Geometry: final body of the model. Coordinates: model frame, mm. Give positions to 0.01 mm unless a question says otherwise; leave off trailing zeros. Write each loop counter-clockwise with the first axis right and the second up, starting at its lowest first coordinate (ties: lowest second). Pieces come first, ordered by that corner, then holes. Notation, with made-up numbers: M 33.25,-8.5 L 86.25,-8.5 A18 cw 86.25,25.5 Z; hole C -3.75,89.25 d11. An arc over 180 degrees is marked long. Answer as a JSON object with one key per item and string values.
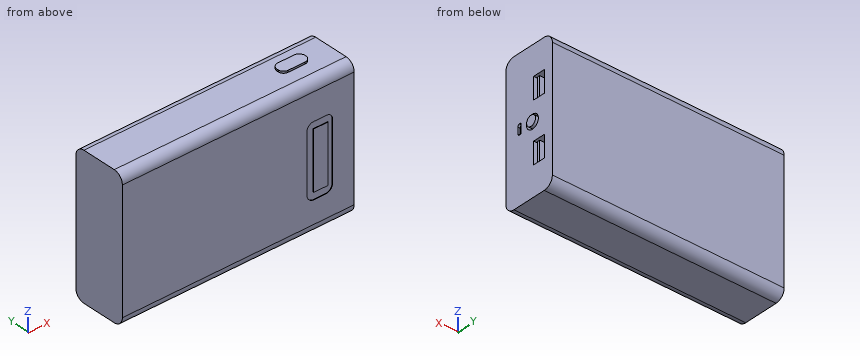
from build123d import *

# Parameters (mm, degrees)
F0_W      = 127
F0_H      = 76.2
F1_DEPTH  = 29.21
F2_R      = 5.08
F3_W      = 6.6195318941
F3_H      = 11.800037697
F4_DEPTH  = 28.956
F5_W      = 1.524
F5_H      = 10.8286906034
F6_DEPTH  = 27.94
F7_R      = 3.7484313793
F8_DEPTH  = 5.588
F9_R      = 2.7812538223
F10_DEPTH = 6.35
F12_DEPTH = 8.636
F14_DEPTH = 7.366
F16_DEPTH = 3.556
F17_DEPTH = 4.572
F18_W     = 7.9864859581
F18_H     = 31.5765572539
F19_DEPTH = 0.254


with BuildPart() as f1:
    # F0 (on Front) → F1 (new body)
    with BuildSketch(Plane.XZ):
        Rectangle(F0_W, F0_H)
    extrude(amount=F1_DEPTH)

    # F2
    f2_edges = [f1.edges().sort_by_distance(p)[0] for p in [
        (0, -29.21, 38.1),
        (0, 0, 38.1),
        (0, -29.21, -38.1),
        (0, 0, -38.1),
    ]]
    fillet(f2_edges, radius=F2_R)

    # F3 (on face) → F4 (cut)
    with BuildSketch(Plane.YZ.offset(63.5)):
        with Locations((-8.3897659471, 16.1171229556)):
            Rectangle(F3_W, F3_H)
        with Locations((-8.3897659471, -16.1171229556)):
            Rectangle(F3_W, F3_H)
    extrude(amount=-F4_DEPTH, mode=Mode.SUBTRACT)

    # F5 (on face) → F6 (join)
    with BuildSketch(Plane.YZ.offset(34.544)):
        with Locations((-9.8508370389, 16.0947965024)):
            Rectangle(F5_W, F5_H)
        with Locations((-9.8508370389, -16.0947965024)):
            Rectangle(F5_W, F5_H)
    extrude(amount=F6_DEPTH)

    # F7 (on face) → F8 (cut)
    with BuildSketch(Plane.YZ.offset(63.5)):
        with Locations((-12.5152766346, -0.14176574)):
            Circle(F7_R)
    extrude(amount=-F8_DEPTH, mode=Mode.SUBTRACT)

    # F9 (on face) → F10 (join)
    with BuildSketch(Plane.YZ.offset(57.912)):
        with Locations((-12.4932004692, -0.0162060605)):
            Circle(F9_R)
    extrude(amount=F10_DEPTH)

    # F11 (on face) → F12 (cut)
    with BuildSketch(Plane.YZ.offset(63.5)):
        with BuildLine():
            Line((-19.6553119308, 2.8573502786), (-20.6747086321, 2.8573502786))
            ThreePointArc((-20.6747086321, 2.8573502786), (-21.4033806509, 2.5555244459), (-21.7052064836, 1.8268524271))
            Line((-21.7052064836, 1.8268524271), (-21.7052064836, -1.6216995807))
            ThreePointArc((-21.7052064836, -1.6216995807), (-21.4033790258, -2.3503755229), (-20.6747030836, -2.6522029807))
            Line((-20.6747030836, -2.6522029807), (-19.6553119308, -2.6522029807))
            Line((-19.6553119308, -2.6522029807), (-19.6553119308, 2.8573502786))
        make_face()
    extrude(amount=-F12_DEPTH, mode=Mode.SUBTRACT)

    # F13 (on face) → F14 (join)
    with BuildSketch(Plane.YZ.offset(54.864)):
        with BuildLine():
            Line((-19.6553119308, -2.6522029807), (-19.6553119308, 2.8573502786))
            Line((-19.6553119308, 2.8573502786), (-20.6747086321, 2.8573502786))
            ThreePointArc((-20.6747086321, 2.8573502786), (-21.4033806509, 2.5555244459), (-21.7052064836, 1.8268524271))
            Line((-21.7052064836, 1.8268524271), (-21.7052064836, -1.6216995807))
            ThreePointArc((-21.7052064836, -1.6216995807), (-21.4033790258, -2.3503755229), (-20.6747030836, -2.6522029807))
            Line((-20.6747030836, -2.6522029807), (-19.6553119308, -2.6522029807))
        make_face()
        Polygon((-20.3632637858, 1.3027831301), (-20.3632637858, 2.1156521834), (-20.0210027397, 2.1156521834), (-20.0210027397, 1.3027831301), (-20.0210027397, 0), (-20.0210027397, -1.7347801622), (-20.3632637858, -1.7347801622), (-20.3632637858, 0), align=None, mode=Mode.SUBTRACT)
    extrude(amount=F14_DEPTH)

    # F15 (on face) → F16 (cut)
    with BuildSketch(Plane.XY.offset(38.1)):
        with BuildLine():
            Line((47.0853128431, -10.2171041071), (38.2701487959, -10.2171041071))
            ThreePointArc((38.2701487959, -10.2171041071), (35.9354614141, -11.1841632846), (34.9684022367, -13.5188506663))
            Line((34.9684022367, -13.5188506663), (34.9684022367, -14.2463892698))
            ThreePointArc((34.9684022367, -14.2463892698), (35.8113644771, -16.2814801432), (37.8464553505, -17.1244423836))
            Line((37.8464553505, -17.1244423836), (47.0853187936, -17.1244423836))
            ThreePointArc((47.0853187936, -17.1244423836), (49.4200057799, -16.15738337), (50.3870647936, -13.8226963836))
            Line((50.3870647936, -13.8226963836), (50.3870647936, -13.5188560576))
            ThreePointArc((50.3870647936, -13.5188560576), (49.4200040371, -11.1841648636), (47.0853128431, -10.2171041071))
        make_face()
    extrude(amount=-F16_DEPTH, mode=Mode.SUBTRACT)

    # F17 (add): a face of the model
    f17_faces = [f1.faces().sort_by_distance(p)[0] for p in [
        (42.6393602825, -13.6846721525, 34.544),
    ]]
    extrude(f17_faces, amount=F17_DEPTH)

    # F18 (on face) → F19 (cut)
    with BuildSketch(Plane.XZ.offset(29.21)):
        with BuildLine():
            Line((48.3708519327, 18.215091899), (41.2623919547, 18.215091899))
            ThreePointArc((41.2623919547, 18.215091899), (38.6504034004, 17.1331708151), (37.5684823165, 14.5211822609))
            Line((37.5684823165, 14.5211822609), (37.5684823165, -16.8614557905))
            ThreePointArc((37.5684823165, -16.8614557905), (38.7072046405, -19.610574669), (41.456323519, -20.749296993))
            Line((41.456323519, -20.749296993), (47.9751093816, -20.749296993))
            ThreePointArc((47.9751093816, -20.749296993), (50.587106677, -19.6673722884), (51.6690313816, -17.055374993))
            Line((51.6690313816, -17.055374993), (51.6690313816, 14.9169124501))
            ThreePointArc((51.6690313816, 14.9169124501), (50.7030169866, 17.249077504), (48.3708519327, 18.215091899))
        make_face()
        with Locations((45.2556349337, -1.2670963661)):
            Rectangle(F18_W, F18_H, mode=Mode.SUBTRACT)
    extrude(amount=-F19_DEPTH, mode=Mode.SUBTRACT)


solid = f1.part
1) Cut plane C-C on y = -7.5. Return loops of the section in (x, z), and give its area (3 significant figures).
Geometry check:
{"outline": "M -63.5,-38.1 L 63.5,-38.1 L 63.5,-22.02 L 34.54,-22.02 L 34.54,-10.22 L 63.5,-10.22 L 63.5,10.22 L 34.54,10.22 L 34.54,22.02 L 63.5,22.02 L 63.5,38.1 L -63.5,38.1 Z", "area": "8,990 mm2"}
2) Contact query for flat-ended pins moving along their axis: P1, Ø6, axis at y = -8.5, z = -24.5, coming from the +X side; P2, Ø9.5, axis at x = 29, y = -11, coming from the +Z side. Output: stop coordinate, or through.
Geometry check:
{"P1": "stops at x = 63.5", "P2": "stops at z = 38.1"}
3) Cut plane B-B on z = 13. Return loops of the section in (x, y), and give its area (3 significant figures).
Geometry check:
{"outline": "M -63.5,-29.21 L 37.57,-29.21 L 37.57,-28.96 L 41.26,-28.96 L 41.26,-29.21 L 49.25,-29.21 L 49.25,-28.96 L 51.67,-28.96 L 51.67,-29.21 L 63.5,-29.21 L 63.5,-11.7 L 34.54,-11.7 L 34.54,-10.61 L 62.48,-10.61 L 62.48,-9.09 L 34.54,-9.09 L 34.54,-5.08 L 63.5,-5.08 L 63.5,0 L -63.5,0 Z", "area": "3,560 mm2"}
4) Cut plane A-A on x = 4.5. Return loops of the section in (y, z).
Geometry check:
{"outline": "M -29.21,-33.02 A5.08 ccw -24.13,-38.1 L -5.08,-38.1 A5.08 ccw 0,-33.02 L 0,33.02 A5.08 ccw -5.08,38.1 L -24.13,38.1 A5.08 ccw -29.21,33.02 Z"}
5) Line query: line 1 (Z direction, x = 44.5, y = -7); line 2 (X direction, y = -8, z = 35); line 3 (Z direction, x = -48, y = -20.5). Output: solid intervals per line, ascending. Write a range as from..to.
Geometry check:
{"line 1": "z = -38.1..-22.02, -10.22..10.22, 22.02..38.1", "line 2": "x = -63.5..63.5", "line 3": "z = -38.1..38.1"}
